```python
from build123d import *

# Parameters (mm, degrees)
F0_R     = 3.175
F1_DEPTH = 3.175
F2_R     = 3.96875
F3_DEPTH = 12.7
F4_R     = 3.175
F5_DEPTH = 3.175
F6_SIZE  = 0.2286


with BuildPart() as f1:
    # F0 (on Top) → F1 (new body)
    with BuildSketch(Plane.XY):
        Circle(F0_R)
    extrude(amount=F1_DEPTH)

    # F2 (on face) → F3 (join)
    with BuildSketch(Plane.XY.offset(3.175)):
        Circle(F2_R)
    extrude(amount=F3_DEPTH)

    # F4 (on face) → F5 (join)
    with BuildSketch(Plane.XY.offset(15.875)):
        Circle(F4_R)
    extrude(amount=F5_DEPTH)

    # F6
    f6_edges = [f1.edges().sort_by_distance(p)[0] for p in [
        (-3.175, 0, 19.05),
        (-3.96875, 0, 15.875),
        (-3.96875, 0, 3.175),
        (-3.175, 0, 0),
    ]]
    chamfer(f6_edges, length=F6_SIZE)


solid = f1.part
```
Geometry: final body of the model. Coordinates: model frame, mm. A direction names the side the tool comes from. Coordinates: 2 decimals unless noted, no trailing zeros. Order: outer loops, then holes, each group sorted by start corner. A loop starts at its lowest first (then second) coordinate and runs counter-clockwise, first axis right, second up. Notation, with made-up numbers: M 72,-29 L 119,-29 A19 ccw 119,7 Z; hole C -6,61.5 d10. An arc over 180 degrees is marked long. Answer in a Markdown table with one row per item. Add a question column.
Q1. Contact query for a flat-ended pin moving along its axis: P1, Ø1.5, axis at y = 2, z = 11.5, coming from the +X side. Output: stop coordinate, or through.
Q2. Reachability of faces 1 (the cylindrical face through (-0.69, -3.1, 1.68)), 2 (the cylindrical face through (-0.69, -3.1, 17.33)), 3 (the flat face through (0, 0, 19.05)) from +Z, -Z, +X, -X, +Y, -Y: full face, straight path, thin tool, end or side. Return the list, or none.
Q3. Section query A-A on x = 0. Return the cut outline in (y, z) (3 decimals), and give its area (3 significant figures).
Q4. Line query: L1, parallel to Z at x = -3.25, y = -1.5 (3 decimals); L2, parallel to Y at x = 2.5, z = 8; L3, parallel to X at y = 0.5, z = 8.5. Output: solid intervals per line, ascending.
Q5. Section query C-C on z = 6.75. Return the cut outline in (x, y), and give its area (3 significant figures).
Completed:
| question | item | result |
|---|---|---|
| 1 | P1 | stops at x = 3.77 |
| 2 | face 1 | -Z |
| 2 | face 2 | +Z |
| 2 | face 3 | +Z, +X, -X, +Y, -Y |
| 3 | outline | M -3.969,3.404 L -3.74,3.175 L -3.175,3.175 L -3.175,0.229 L -2.946,0 L 2.946,0 L 3.175,0.229 L 3.175,3.175 L 3.74,3.175 L 3.969,3.404 L 3.969,15.646 L 3.74,15.875 L 3.175,15.875 L 3.175,18.821 L 2.946,19.05 L -2.946,19.05 L -3.175,18.821 L -3.175,15.875 L -3.74,15.875 L -3.969,15.646 Z |
| 3 | area | 141 mm2 |
| 4 | L1 | z = 3.175 to 15.875 |
| 4 | L2 | y = -3.08 to 3.08 |
| 4 | L3 | x = -3.94 to 3.94 |
| 5 | outline | C 0,0 d7.94 |
| 5 | area | 49.5 mm2 |
